Source: CAD feature listing. Evaluate the final solid. Frame: model axes, mm. Coordinates: 2 decimals unless noted, no trailing zeros. Loops run counter-clockwise (first coordinate to the right, second up) from the corner with the lowest first, then second, coordinate; pieces in that order, holes last.
Item 1: Section query C-C, the plane y = 7. Return the cut outline in (x, z) (1 decimal), then the cut area to 3 significant figures.
Item 2: Section query B-B, the plane x = 0. Return the cut outline in (y, z), then the cut area to 3 significant figures.
Item 3: Pin query (flat end, axial travel): pin 1 Ø15 at (x, z) = (0, 0) entering from -Y. Return the tip coordinate at first contact, or that it passes through.
Item 4: Line query: probe 1 along X at (y, z) = (1.05, 0); probe 2 along X at (y, z) = (9.25, 0); probe 3 along Y at (x, z) = (16, 4.5). Output: solid intervals per line, ascending.
Item 5: Section query D-D, the plane z = -15.5. Return the cut outline in (x, y), then the cut area to 3 significant figures.
Item 6: Section query A-A, the plane z = 0. Return the cut outline in (x, y), then the cut area to 3 significant figures.
```python
from build123d import *

# Parameters (mm, degrees)
SKETCH1_W           = 279.4
SKETCH1_H           = 50.8
BOSS_EXTRUDE1_DEPTH = 12.7
SKETCH2_R           = 20.6375
CUT_EXTRUDE1_DEPTH  = 11.1125
SKETCH3_R           = 12.7
CUT_EXTRUDE2_DEPTH  = 143.42449809


with BuildPart() as part:
    # Sketch1 → Boss-Extrude1 (new body)
    with BuildSketch(Plane(origin=(0, 0, 0), x_dir=(1, 0, 0), z_dir=(0, 1, 0))):
        Rectangle(SKETCH1_W, SKETCH1_H)
    extrude(amount=BOSS_EXTRUDE1_DEPTH)

    # Sketch2 → Cut-Extrude1 (cut)
    with BuildSketch(Plane(origin=(0, 12.7, 0), x_dir=(1, 0, 0), z_dir=(0, 1, 0))):
        with Locations(Location((0, 0, 0), (0, 0, 270))):
            Circle(SKETCH2_R)
    extrude(amount=-CUT_EXTRUDE1_DEPTH, mode=Mode.SUBTRACT)

    # Sketch3 → Cut-Extrude2 (cut, through all)
    with BuildSketch(Plane(origin=(0, 1.5875, 0), x_dir=(1, 0, 0), z_dir=(0, 1, 0))):
        with Locations(Location((0, 0, 0), (0, 0, 270))):
            Circle(SKETCH3_R)
    extrude(amount=-CUT_EXTRUDE2_DEPTH, mode=Mode.SUBTRACT)


solid = part.part
```
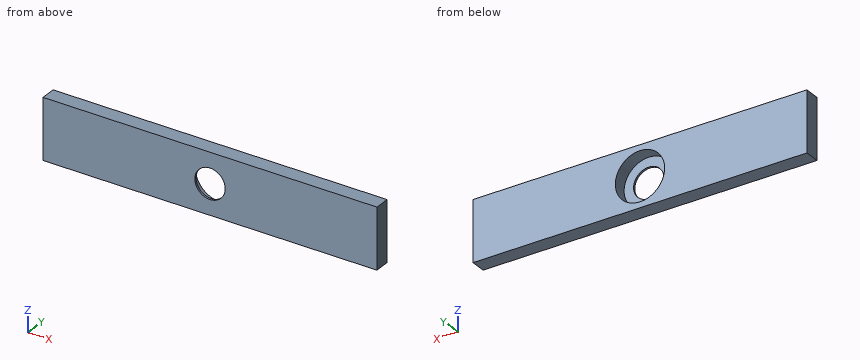
Verdict:
1. outline: (-139.7, -25.4) - (139.7, -25.4) - (139.7, 25.4) - (-139.7, 25.4) - close; hole circle Ø41.3 at (0, 0)
1. area: 12,900 mm2
2. outline: (0, -25.4) - (12.7, -25.4) - (12.7, -20.64) - (1.59, -20.64) - (1.59, -12.7) - (0, -12.7) - close; (0, 12.7) - (1.59, 12.7) - (1.59, 20.64) - (12.7, 20.64) - (12.7, 25.4) - (0, 25.4) - close
2. area: 146 mm2
3. pin 1: passes through
4. probe 1: x = -139.7 to -12.7, 12.7 to 139.7
4. probe 2: x = -139.7 to -20.64, 20.64 to 139.7
4. probe 3: y = 0 to 1.59
5. outline: (-139.7, 0) - (139.7, 0) - (139.7, 12.7) - (13.63, 12.7) - (13.63, 1.59) - (-13.63, 1.59) - (-13.63, 12.7) - (-139.7, 12.7) - close
5. area: 3,250 mm2
6. outline: (-139.7, 0) - (-12.7, 0) - (-12.7, 1.59) - (-20.64, 1.59) - (-20.64, 12.7) - (-139.7, 12.7) - close; (12.7, 0) - (139.7, 0) - (139.7, 12.7) - (20.64, 12.7) - (20.64, 1.59) - (12.7, 1.59) - close
6. area: 3,050 mm2
